```python
from build123d import *

# Parameters (mm, degrees)
SKETCH1_W           = 82
SKETCH1_H           = 40
SKETCH1_R           = 2
SKETCH1_W_2         = 12.5
BOSS_EXTRUDE1_DEPTH = 3
BOSS_EXTRUDE2_DEPTH = 42.5
CUT_EXTRUDE1_DEPTH  = 88.459990853
SKETCH4_R           = 12
SKETCH4_R_2         = 1.65
CUT_EXTRUDE2_DEPTH  = 102.95219468
SKETCH7_W           = 25
SKETCH7_H           = 5
BOSS_EXTRUDE3_DEPTH = 20
BOSS_EXTRUDE4_REACH = 102.649
SKETCH7_3_W         = 25
SKETCH7_3_H         = 5
CUT_EXTRUDE3_DEPTH  = 99.459382488
CUT_EXTRUDE4_DEPTH  = 91.32856691


with BuildPart() as part:
    # Sketch1 → Boss-Extrude1 (new body)
    # profile 1 of 2: a face of its own
    with BuildSketch(Plane(origin=(0, 0, 0), x_dir=(1, 0, 0), z_dir=(0, 1, 0))):
        with Locations((41, 20)):
            Rectangle(SKETCH1_W, SKETCH1_H)
        with Locations(Location((78, 23.86, 0), (0, 0, 270))):
            Circle(SKETCH1_R, mode=Mode.SUBTRACT)
        with Locations(Location((78, 5, 0), (0, 0, 270))):
            Circle(SKETCH1_R, mode=Mode.SUBTRACT)
    # profile 2 of 2: a face of its own
    with BuildSketch(Plane(origin=(0, 0, 0), x_dir=(1, 0, 0), z_dir=(0, 1, 0))):
        with Locations((-6.25, 20)):
            Rectangle(SKETCH1_W_2, SKETCH1_H)
        with Locations(Location((-7.5, 5, 0), (0, 0, 270))):
            Circle(SKETCH1_R, mode=Mode.SUBTRACT)
        with Locations(Location((-7.5, 23.86, 0), (0, 0, 270))):
            Circle(SKETCH1_R, mode=Mode.SUBTRACT)
    extrude(amount=BOSS_EXTRUDE1_DEPTH)

    # Sketch2 → Boss-Extrude2 (add)
    with BuildSketch(Plane(origin=(0, 3, 0), x_dir=(1, 0, 0), z_dir=(0, 1, 0))):
        Polygon((10, 2.5), (10, 40), (8, 40), (8, 0), (54.5, 0), (54.5, 40), (52.5, 40), (52.5, 2.5), align=None)
    extrude(amount=BOSS_EXTRUDE2_DEPTH)

    # Sketch3 → Cut-Extrude1 (cut, through all)
    with BuildSketch(Plane(origin=(54.5, 6, 0), x_dir=(0, 0, -1), z_dir=(-1, 0, 0))):
        Polygon((2.5, -39.5), (40, -39.5), (40, 3), align=None)
    extrude(amount=CUT_EXTRUDE1_DEPTH, mode=Mode.SUBTRACT)

    # Sketch4 → Cut-Extrude2 (cut, through all)
    with BuildSketch(Plane.XY):
        with Locations((31.25, 24.25)):
            Circle(SKETCH4_R)
        with Locations((16.25, 9.25)):
            Circle(SKETCH4_R_2)
        with Locations((16.25, 39.25)):
            Circle(SKETCH4_R_2)
        with Locations((46.25, 39.25)):
            Circle(SKETCH4_R_2)
        with Locations((46.25, 9.25)):
            Circle(SKETCH4_R_2)
    extrude(amount=-CUT_EXTRUDE2_DEPTH, mode=Mode.SUBTRACT)

    # Sketch7 → Boss-Extrude3 (add)
    with BuildSketch(Plane(origin=(0, 3, 0), x_dir=(1, 0, 0), z_dir=(0, 1, 0))):
        with Locations((67, 32.5)):
            Rectangle(SKETCH7_W, SKETCH7_H)
    extrude(amount=BOSS_EXTRUDE3_DEPTH)

    # Boss-Extrude4: up to this plane
    boss_extrude4_end = Plane(origin=(-12.5, 21.157587549, -23.978599222), z_dir=(0, -0.6616216370868465, 0.7498378553650924))
    # Sketch7_3 → Boss-Extrude4 (add, up to the surface)
    with BuildSketch(Plane(origin=(0, 3, 0), x_dir=(1, 0, 0), z_dir=(0, 1, 0)), mode=Mode.PRIVATE) as boss_extrude4_sk1:
        with Locations((67, 12.5)):
            Rectangle(SKETCH7_3_W, SKETCH7_3_H)
    boss_extrude4_tool1 = split(extrude(boss_extrude4_sk1.sketch, amount=BOSS_EXTRUDE4_REACH, mode=Mode.PRIVATE), bisect_by=boss_extrude4_end, keep=Keep.BOTH, mode=Mode.PRIVATE)
    add(boss_extrude4_tool1.solids().sort_by_distance((67, 3, -12.5))[0])

    # Sketch9 → Cut-Extrude3 (cut, through all)
    with BuildSketch(Plane.XY.offset(-10)):
        with BuildLine():
            Line((64.330095427, 13.170078856), (64.330095427, 5.052055091))
            ThreePointArc((64.330095427, 5.052055091), (62.856131757, 3.578091421), (61.382168087, 5.052055091))
            Line((61.382168087, 5.052055091), (61.382168087, 13.170078856))
            ThreePointArc((61.382168087, 13.170078856), (62.856131757, 14.644042526), (64.330095427, 13.170078856))
        make_face()
        with BuildLine():
            Line((69.669904573, 13.170078856), (69.669904573, 5.052055091))
            ThreePointArc((69.669904573, 5.052055091), (71.143868243, 3.578091421), (72.617831913, 5.052055091))
            Line((72.617831913, 5.052055091), (72.617831913, 13.170078856))
            ThreePointArc((72.617831913, 13.170078856), (71.143868243, 14.644042526), (69.669904573, 13.170078856))
        make_face()
    extrude(amount=-CUT_EXTRUDE3_DEPTH, mode=Mode.SUBTRACT)

    # Sketch11 → Cut-Extrude4 (cut, through all)
    with BuildSketch(Plane.ZY.offset(-54.5)):
        Polygon((-35, 17.332602518), (-30, 23), (-35, 23), align=None)
    extrude(amount=-CUT_EXTRUDE4_DEPTH, mode=Mode.SUBTRACT)


solid = part.part
```
Design review of the part built by this model. Coordinates are the model's own, in mm. A direction names the side the tool comes from. Give positions to 0.01 mm unless a question says otherwise; leave off trailing zeros. Order: outer loops, then holes, each group sorted by start corner. A loop starts at its lowest first (then second) coordinate and runs counter-clockwise, first axis right, second up. Notation, with made-up numbers: (-11.75, 44) -> (36.25, 44) arc R28 cw to (36.25, 78) -> close; hole circle Ø9 at (65.25, 87.5). An arc over 180 degrees is marked (long way). Write item = value, one per line. Start each with the question number.
(1) We need section D-D on z = -23.86. Write out the cut boundary in (x, y), plus the area to 3 significant figures.
(2) We need section A-A on x = 16.25. Write out the cut boundary in (y, z), plus the area to 3 significant figures.
(3) To check wall thickness, follow line 1 along X through (y, z) = (1.5, -23.86); line 2 along X through (y, z) = (9, -1); line 3 along X through (y, z) = (10.5, -15.5). State the ranges of each line that lie inside material, in increasing order.
(4) Mouldability with a two-part tool opening along Y and no side actions: class faces 4 (the face through (34, 0, -20)), 5 (the face through (72.618, 9, -32)), 6 (the face through (54.5, 5, -37)) as +Y half, -Y half, draft (parallel to the pull), parting line (faces both ways), or undercut.
(5) For faces 1 (the face through (71.11, 3.58, -32.47)), 2 (the face through (79.5, 11, -32)), 3 (the face through (8, 19, -16)), list the 3-axis set-ups (+Z, -Z, +X, -X, +Y, -Y) from which the entire face can be reached by the end or side of a thin tool; tool diameter is ignored.
(6) For pin 1 (1.5 mm diameter, centred on y = 8.5, z = -13.5, fed in from +X); pin 2 (1.5 mm diameter, centred on x = 0.5, z = -20, fed in from +Y); pin 3 (8 mm diameter, centred on y = 28.5, z = -28, fed in from -X); pin 4 (4.5 mm diameter, centred on x = 69, y = 9.5, fed in from -Z), all flat-tipped, find the tip position at first contact; note any pin that passes through.
(7) We need section C-C on y = 24.25. Write out the cut boundary in (x, z), plus the area to 3 significant figures.
(8) We need section B-B on x = 31.25. Write out the cut boundary in (y, z).
Numbers:
q1.outline = (-12.5, 0) -> (-9.5, 0) -> (-9.5, 3) -> (-12.5, 3) -> close; (-5.5, 0) -> (76, 0) -> (76, 3) -> (54.5, 3) -> (54.5, 21.29) -> (52.5, 21.29) -> (52.5, 3) -> (10, 3) -> (10, 21.29) -> (8, 21.29) -> (8, 3) -> (-5.5, 3) -> close; (80, 0) -> (82, 0) -> (82, 3) -> (80, 3) -> close
q1.area = 333 mm^2
q2.outline = (0, -40) -> (3, -40) -> (3, -2.5) -> (7.6, -2.5) -> (7.6, 0) -> (0, 0) -> close; (10.9, -2.5) -> (37.6, -2.5) -> (37.6, 0) -> (10.9, 0) -> close; (40.9, -2.5) -> (45.5, -2.5) -> (45.5, 0) -> (40.9, 0) -> close
q2.area = 210 mm^2
q3.line_1 = -12.5 to -9.5, -5.5 to 76, 80 to 82
q3.line_2 = 8 to 14.62, 17.88 to 44.62, 47.88 to 54.5
q3.line_3 = 8 to 10, 52.5 to 54.5
q4.face_4 = -Y half
q4.face_5 = undercut
q4.face_6 = draft
q5.face_1 = +Z, -Z
q5.face_2 = +Z, -Z, +X, +Y
q5.face_3 = +Z, -Z, -X, +Y
q6.pin_1 = 79.5
q6.pin_2 = 3
q6.pin_3 = through
q6.pin_4 = -35
q7.outline = (8, -21.25) -> (10, -21.25) -> (10, -2.5) -> (19.25, -2.5) -> (19.25, 0) -> (8, 0) -> close; (43.25, -2.5) -> (52.5, -2.5) -> (52.5, -21.25) -> (54.5, -21.25) -> (54.5, -15) -> (79.5, -15) -> (79.5, -10) -> (54.5, -10) -> (54.5, 0) -> (43.25, 0) -> close
q7.area = 256 mm^2
q8.outline = (0, -40) -> (3, -40) -> (3, -2.5) -> (12.25, -2.5) -> (12.25, 0) -> (0, 0) -> close; (36.25, -2.5) -> (45.5, -2.5) -> (45.5, 0) -> (36.25, 0) -> close
